Model file for the job. Use its own axes, mm. A direction names the side the tool comes from. Round coordinates to 2 decimals unless told otherwise and drop trailing zeros. Order: outer loops, then holes, each group sorted by start corner. A loop starts at its lowest first (then second) coordinate and runs counter-clockwise, first axis right, second up. Notation, with made-up numbers: M 87.25,-31 L 114.25,-31 A17 cw 114.25,-5 Z; hole C 3,-19 d5. An arc over 180 degrees is marked long. Return JSON: item names as keys, results as strings. Group by question number.
Item 1: Pull direction X, two halves, no side cores. Call faces 4 (the face through (68.78, 9.5, -51.25)), 5 (the face through (-72.34, 6.26, -52.4)), 6 (the face through (-61, 0, -67)): pulls with the +X half, pulls with the -X half, needs draft (parallel to the pull), parting line crosses it, or undercut.
Item 2: Slice it at A-A on z = -102.8. Write the cut outline in (x, y) (3 decimals).
Item 3: Which spindle directions (+Z, -Z, +X, -X, +Y, -Y) get a long thin tool onto all of the face, cutting with end or side? Do faces 1 (the face through (58.05, 6.44, -50.96)), 2 (the face through (-59, 12.7, -58)), 3 (the face through (-64, 6.2, -58)). Say none if no direction does.
Item 4: Pin check, flat tips, straight feed: pin 1 Ø5.5 at (x, z) = (54, -1) entering from +Y; pin 2 Ø3 at (y, z) = (1.5, -87) entering from -X; pin 3 Ø3 at (y, z) = (9, -65) entering from +X. Stop position of each tip, or through.
Item 5: Slice it at C-C on z = 15. Write the cut outline in (x, y), then the cut area to 3 significant figures.
Item 6: Slice it at B-B on x = 20. Write the cut outline in (y, z).
Item 7: Probe line 1 along Z through (x, y) = (-35, 9.75); line 2 along X through (y, z) = (7.5, -89); line 3 along X through (y, z) = (6.5, -21.5). List the from-to ranges inside material, lowest first.
from build123d import *

# Parameters (mm, degrees)
SKETCH1_R           = 40
SKETCH1_R_2         = 50.8
SKETCH1_R_3         = 5.75
BOSS_EXTRUDE1_DEPTH = 12.7
SKETCH10_R          = 3.175
CUT_EXTRUDE6_DEPTH  = 194.127134292
SKETCH12_R          = 5.5
CUT_EXTRUDE8_DEPTH  = 3
CUT_EXTRUDE9_DEPTH  = 6.5
CUT_EXTRUDE10_DEPTH = 194.127134292
FILLET1_R           = 3
FILLET2_R           = 3


with BuildPart() as part:
    # Sketch1 → Boss-Extrude1 (new body)
    with BuildSketch(Plane(origin=(0, 0, 0), x_dir=(1, 0, 0), z_dir=(0, 1, 0))):
        with BuildLine():
            Line((-74.704056398, 99.012658228), (-69.910213207, 4.455696203))
            ThreePointArc((-69.910213207, 4.455696203), (0, -62), (69.910213207, 4.455696203))
            Line((69.910213207, 4.455696203), (74.704056398, 99.012658228))
            ThreePointArc((74.704056398, 99.012658228), (0, 177.6), (-74.704056398, 99.012658228))
        make_face()
        with Locations(Location((0, 0, 0), (0, 0, 270))):
            Circle(SKETCH1_R, mode=Mode.SUBTRACT)
        with Locations(Location((0, 102.8, 0), (0, 0, 270))):
            Circle(SKETCH1_R_2, mode=Mode.SUBTRACT)
        with Locations(Location((40.163665171, 142.963665171, 0), (0, 0, 270))):
            Circle(SKETCH1_R_3, mode=Mode.SUBTRACT)
        with Locations(Location((40.163665171, 62.636334829, 0), (0, 0, 270))):
            Circle(SKETCH1_R_3, mode=Mode.SUBTRACT)
        with Locations(Location((-40.163665171, 62.636334829, 0), (0, 0, 270))):
            Circle(SKETCH1_R_3, mode=Mode.SUBTRACT)
        with Locations(Location((-40.163665171, 142.963665171, 0), (0, 0, 270))):
            Circle(SKETCH1_R_3, mode=Mode.SUBTRACT)
    extrude(amount=BOSS_EXTRUDE1_DEPTH)

    # Sketch10 → Cut-Extrude6 (cut, through all)
    with BuildSketch(Plane(origin=(0, 12.7, 0), x_dir=(1, 0, 0), z_dir=(0, 1, 0))):
        with Locations(Location((-52, 0, 0), (0, 0, 270))):
            Circle(SKETCH10_R)
        with Locations(Location((-60.8, 102.8, 0), (0, 0, 270))):
            Circle(SKETCH10_R)
        with Locations(Location((60.8, 102.8, 0), (0, 0, 90))):
            Circle(SKETCH10_R)
        with Locations(Location((52, 0, 0), (0, 0, 90))):
            Circle(SKETCH10_R)
    extrude(amount=-CUT_EXTRUDE6_DEPTH, mode=Mode.SUBTRACT)

    # Sketch12 → Cut-Extrude8 (cut)
    with BuildSketch(Plane(origin=(0, 12.7, 0), x_dir=(1, 0, 0), z_dir=(0, 1, 0))):
        with Locations(Location((-60.8, 102.8, 0), (0, 0, 270))):
            Circle(SKETCH12_R)
        with Locations(Location((60.8, 102.8, 0), (0, 0, 270))):
            Circle(SKETCH12_R)
        with Locations(Location((52, 0, 0), (0, 0, 270))):
            Circle(SKETCH12_R)
        with Locations(Location((-52, 0, 0), (0, 0, 270))):
            Circle(SKETCH12_R)
    extrude(amount=-CUT_EXTRUDE8_DEPTH, mode=Mode.SUBTRACT)

    # Sketch13 → Cut-Extrude9 (cut)
    with BuildSketch(Plane(origin=(0, 12.7, 0), x_dir=(1, 0, 0), z_dir=(0, 1, 0))):
        with BuildLine():
            Line((-71.208545738, 99.189873418), (-66.414702546, 4.632911392))
            ThreePointArc((-66.414702546, 4.632911392), (0, -58.5), (66.414702546, 4.632911392))
            Line((66.414702546, 4.632911392), (71.208545738, 99.189873418))
            ThreePointArc((71.208545738, 99.189873418), (0, 174.1), (-71.208545738, 99.189873418))
        make_face()
        with BuildLine():
            Line((-65.515856948, 99.478481013), (-60.722013757, 4.921518987))
            ThreePointArc((-60.722013757, 4.921518987), (0, -52.8), (60.722013757, 4.921518987))
            Line((60.722013757, 4.921518987), (65.515856948, 99.478481013))
            ThreePointArc((65.515856948, 99.478481013), (0, 168.4), (-65.515856948, 99.478481013))
        make_face(mode=Mode.SUBTRACT)
    extrude(amount=-CUT_EXTRUDE9_DEPTH, mode=Mode.SUBTRACT)

    # Sketch14 → Cut-Extrude10 (cut, through all)
    with BuildSketch(Plane(origin=(0, 12.7, 0), x_dir=(1, 0, 0), z_dir=(0, 1, 0))):
        with BuildLine():
            Line((-60.247807343, 94.317955242), (-55.850268123, 7.577957204))
            ThreePointArc((-55.850268123, 7.577957204), (-43.603288319, 1.321072649), (-53.33734455, -8.394135426))
            ThreePointArc((-53.33734455, -8.394135426), (-33.157557534, -36.880022041), (0, -47.8))
            ThreePointArc((0, -47.8), (33.157557534, -36.880022041), (53.33734455, -8.394135426))
            ThreePointArc((53.33734455, -8.394135426), (43.603288319, 1.321072649), (55.850268123, 7.577957204))
            Line((55.850268123, 7.577957204), (60.247807343, 94.317955242))
            ThreePointArc((60.247807343, 94.317955242), (52.300864134, 102.678799624), (60.006167763, 111.262850015))
            ThreePointArc((60.006167763, 111.262850015), (39.746139995, 148.544992682), (0, 163.4))
            ThreePointArc((0, 163.4), (-39.746139995, 148.544992682), (-60.006167763, 111.262850015))
            ThreePointArc((-60.006167763, 111.262850015), (-52.300864134, 102.678799624), (-60.247807343, 94.317955242))
        make_face()
    extrude(amount=-CUT_EXTRUDE10_DEPTH, mode=Mode.SUBTRACT)

    # Fillet1
    fillet1_edges = [part.edges().sort_by_distance(p)[0] for p in [
        (-60.006167763, 6.35, -111.262850015),
        (-53.33734455, 6.35, 8.394135426),
        (-55.850268123, 6.35, -7.577957204),
        (-60.247807343, 6.35, -94.317955242),
        (60.006167763, 6.35, -111.262850015),
        (60.247807343, 6.35, -94.317955242),
        (55.850268123, 6.35, -7.577957204),
        (53.33734455, 6.35, 8.394135426),
    ]]
    fillet(fillet1_edges, radius=FILLET1_R)

    # Fillet2
    fillet2_edges = [part.edges().sort_by_distance(p)[0] for p in [
        (-39.585032528, 6.35, -148.684476675),
        (-45.884476675, 6.35, -142.385032528),
        (39.585032528, 6.35, -148.684476675),
        (45.884476675, 6.35, -142.385032528),
    ]]
    fillet(fillet2_edges, radius=FILLET2_R)


solid = part.part
Output values:
{
 "1": {"face 4": "undercut", "face 5": "pulls with the -X half", "face 6": "needs draft"},
 "2": {"outline": "M -74.8,0 L -63.975,0 L -63.975,9.7 L -65.6,9.7 L -65.6,6.2 L -71.3,6.2 L -71.3,12.7 L -74.8,12.7 Z; M -57.625,0 L -52.3,0 L -52.3,12.7 L -55.3,12.7 L -55.3,9.7 L -57.625,9.7 Z; M 52.3,0 L 57.625,0 L 57.625,9.7 L 55.3,9.7 L 55.3,12.7 L 52.3,12.7 Z; M 63.975,0 L 74.8,0 L 74.8,12.7 L 71.3,12.7 L 71.3,6.2 L 65.6,6.2 L 65.6,9.7 L 63.975,9.7 Z"},
 "3": {"face 1": "+Y, -Y", "face 2": "+Z, -Z, +X, -X, +Y", "face 3": "+Y"},
 "4": {"pin 1": "y = 9.7", "pin 2": "x = -74.17", "pin 3": "x = 73.06"},
 "5": {"outline": "M -66.11,0 L -50.84,0 L -50.84,12.7 L -56.28,12.7 L -56.28,6.2 L -62.4,6.2 L -62.4,12.7 L -66.11,12.7 Z; M 50.84,0 L 66.11,0 L 66.11,12.7 L 62.4,12.7 L 62.4,6.2 L 56.28,6.2 L 56.28,12.7 L 50.84,12.7 Z", "area": "308 mm²"},
 "6": {"outline": "M 0,-174.88 L 12.7,-174.88 L 12.7,-171.24 L 6.2,-171.24 L 6.2,-165.28 L 12.7,-165.28 L 12.7,-160 L 0,-160 Z; M 0,44.09 L 12.7,44.09 L 12.7,49.42 L 6.2,49.42 L 6.2,55.42 L 12.7,55.42 L 12.7,59.08 L 0,59.08 Z"},
 "7": {"line 1": "-168.91 to -164.92, -158.28 to -152.27, 35.46 to 41.72, 48.54 to 52.62", "line 2": "-74.2 to -70.69, -64.98 to -59.98, 59.98 to 64.98, 70.69 to 74.2", "line 3": "-70.77 to -67.27, -61.56 to -56.56, 56.56 to 61.56, 67.27 to 70.77"}
}
